Autodesk Inventor part; units mm, degrees
ref_plane "YZ Plane" through (0, 0, 0) normal (1, 0, 0) x (0, 1, 0)
ref_plane "XZ Plane" through (0, 0, 0) normal (0, 1, 0) x (-1, 0, 0)
ref_plane "XY Plane" through (0, 0, 0) normal (0, 0, 1) x (1, 0, 0)
sketch "スケッチ1" plane through (0, 0, 0) normal (0, 1, 0) x (-1, 0, 0)
  line L0 (0, 0) -> (40, 0)
  line L1 (40, 0) -> (40, -50)
  line L2 (40, -50) -> (0, -50)
  line L3 (0, -50) -> (0, 0)
  line L4 (35, -50) -> (35, 0)
  line L5 (30, -50) -> (30, 0)
  line L6 (25, -50) -> (25, 0)
  line L7 (20, -50) -> (20, 0)
  line L8 (15, -50) -> (15, 0)
  line L9 (10, -50) -> (10, 0)
  line L10 (5, -50) -> (5, 0)
  dimension "d0" = 40
  dimension "d1" = 50
  dimension "d2" = 5
  dimension "d6" = 5
extrude "押し出し1" add sketch "スケッチ1" along normal blind 5
sketch "スケッチ4" plane through (0, 0, 0) normal (0, -1, 0) x (1, 0, 0)
  line L0 (-40, -50) -> (-40, 0)
  line L1 (-40, -17.5) -> (0, -17.5)
  line L2 (0, 0) -> (0, -50)
  line L3 (0, -32.5) -> (-35, -32.5)
  line L4 (-40, 0) -> (0, 0)
  line L5 (0, -50) -> (-40, -50)
  line L6 (-25, -50) -> (-25, 0)
  line L7 (-20, -50) -> (-20, 0)
  line L8 (-15, -50) -> (-15, 0)
  line L9 (-40, -25) -> (0, -25)
  point P0 (-25, -17.5)
  point P1 (-15, -17.5)
  point P2 (-15, -32.5)
  point P3 (-25, -32.5)
  dimension "d49" = 15
  dimension "d50" = 15
hole "穴3" at (-15, 0, -17.5) at (-15, 0, -32.5) at (-25, 0, -17.5) at (-25, 0, -32.5) direction (0, 1, 0) diameter 3.1 end through all
sketch "スケッチ5" plane through (0, 0, -50) normal (0, 0, -1) x (-1, 0, 0)
  line L0 (40, 0) -> (40, 5)
  line L1 (40, 2.5) -> (0, 2.5)
  line L2 (0, 0) -> (0, 5)
  point P0 (35, 0)
  point P1 (35, 0)
  point P2 (35, 0)
  point P3 (5, 0)
  point P4 (5, 0)
  point P5 (5, 0)
  point P6 (35, 2.5)
  point P7 (5, 2.5)
hole "穴4" at (-35, 2.5, -50) at (-5, 2.5, -50) direction (0, 0, 1) diameter 2.5 end through all
sketch "スケッチ6" plane through (0, 5, 0) normal (0, 1, 0) x (1, 0, 0)
  line L0 (-40, 0) -> (0, 0)
  line L1 (-35, 0) -> (-35, 50)
  line L2 (-6.25, 0) -> (-6.25, 50)
  circle A0 centre (-15, 32.5) radius 1.55
  circle A1 centre (-25, 32.5) radius 1.55
  point P0 (-35, 32.5)
  point P1 (-35, 17.5)
  dimension "d52" = 15
  dimension "d60" = 10
hole "穴5" at (-35, 5, -32.5) at (-35, 5, -17.5) direction (0, -1, 0) diameter 3.1 end through all
properties part number "hand2_11" material "アルミニウム 6061-AHC"
Design review of the part built by this model. Coordinates are the model's own, in mm. Round coordinates to 2 decimals unless told otherwise and drop trailing zeros. Loops run counter-clockwise (first coordinate to the right, second up) from the corner with the lowest first, then second, coordinate; pieces in that order, holes last. Notation, with made-up numbers: M 20,81.5 L 62,81.5 A14 ccw 62,85.5 Z; hole C -0.5,9 d1. An arc over 180 degrees is marked long. Answer as a JSON object with one key per item and string values.
Item 1: The part is to be moulded in two halves that separate along Z. For faces 1 (the flat face through (-20, 5, -25)), 2 (the flat face through (-20, 2, -50)), 3 (the cylindrical face through (-16.537, 2.535, -17.298)), say which applies: pulls with the +Z half, pulls with the -Z half, needs draft (parallel to the pull), parting line crosses it, or undercut.
Answer sheet:
{"face 1": "needs draft", "face 2": "pulls with the -Z half", "face 3": "undercut"}
Item 2: We need section D-D on x = -35. Give the boundary of the cut face in (y, z).
Answer sheet:
{"outline": "M 0,-50 L 1.25,-50 L 1.25,-34.05 L 0,-34.05 Z; M 0,-30.95 L 1.25,-30.95 L 1.25,-19.05 L 0,-19.05 Z; M 0,-15.95 L 1.25,-15.95 L 1.25,0 L 0,0 Z; M 3.75,-50 L 5,-50 L 5,-34.05 L 3.75,-34.05 Z; M 3.75,-30.95 L 5,-30.95 L 5,-19.05 L 3.75,-19.05 Z; M 3.75,-15.95 L 5,-15.95 L 5,0 L 3.75,0 Z"}
Item 3: Clearance check with a flat-ended pin moving along its axis: P1, Ø1.5, axis at y = 1, z = -40, coming from the +X side. State where the tip first meets the part, or that it passes through.
Answer sheet:
{"P1": "stops at x = 0"}
Item 4: We need section A-A on y = 2.5. Give the boundary of the cut face in (x, z).
Answer sheet:
{"outline": "M -40,-50 L -36.25,-50 L -36.25,-33.42 A1.55 cw -36.25,-31.58 L -36.25,-18.42 A1.55 cw -36.25,-16.58 L -36.25,0 L -40,0 Z; M -33.75,-50 L -6.25,-50 L -6.25,0 L -33.75,0 L -33.75,-16.58 A1.55 cw -33.75,-18.42 L -33.75,-31.58 A1.55 cw -33.75,-33.42 Z; M -3.75,-50 L 0,-50 L 0,0 L -3.75,0 Z; hole C -25,-32.5 d3.1; hole C -25,-17.5 d3.1; hole C -15,-32.5 d3.1; hole C -15,-17.5 d3.1"}
Item 5: We need section C-C on x = -25. Give the boundary of the cut face in (y, z).
Answer sheet:
{"outline": "M 0,-50 L 5,-50 L 5,-34.05 L 0,-34.05 Z; M 0,-30.95 L 5,-30.95 L 5,-19.05 L 0,-19.05 Z; M 0,-15.95 L 5,-15.95 L 5,0 L 0,0 Z"}
Item 6: Wall thickness on L1, parallel to X at y = 2.5, z = -29; L2, parallel to X at y = 4, z = -32.5; L3, parallel to Z at x = -25, y = 2.85: over which ranges is each line inside the solid? List them lowest first. Write a range as from..to.
Answer sheet:
{"L1": "x = -40..-36.25, -33.75..-6.25, -3.75..0", "L2": "x = -40..-36.55, -33.45..-26.55, -23.45..-16.55, -13.45..0", "L3": "z = -50..-34.05, -30.95..-19.05, -15.95..0"}
Item 7: We need section B-B on z = -17.5. Give the boundary of the cut face in (x, y), and give its area (3 significant figures).
Answer sheet:
{"outline": "M -40,0 L -36.55,0 L -36.55,5 L -40,5 Z; M -33.45,0 L -26.55,0 L -26.55,5 L -33.45,5 Z; M -23.45,0 L -16.55,0 L -16.55,5 L -23.45,5 Z; M -13.45,0 L 0,0 L 0,5 L -13.45,5 Z; hole C -5,2.5 d2.5", "area": "149 mm^2"}
